Answer from the drawing. Dimensions are ordinates in mm from the lowest x, y and z of the part. A direction names the side the tool comes from. Give positions to 0.01 mm unless a question says otherwise; leave off trailing zeros. Loops run counter-clockwise (first coordinate to the right, second up) from the corner with the lowest first, then second, coordinate; pieces in that order, holes last. Notation, with made-up numbers: (-8, 45.5) - (47, 45.5) arc R15 ccw to (47, 69.5) - close; hole circle Ø9 at (20, 69). An arc over 180 degrees is marked (long way). Answer as CSV lines item,"result". Start each with the question number.
1) Flat-ended cylindrical pins translate along their axes: pin 1 (1.5 mm diameter, centred on x = 3.5, y = 1.5, fed in from +Z); pin 2 (1.5 mm diameter, centred on y = 5, z = 6.5, fed in from -X); pin 3 (1 mm diameter, centred on y = 1.5, z = 3, fed in from -X). Find the tip coordinate at first contact, or state that the pin passes through.
2) A cutting plane is placed at B-B (x = 10). Determine the outline of the cut face in (y, z), and give its area (3 significant figures).
3) For a pull along X with two mould halves and no side action, classify the marked faces 1, 2 and 3 as pulls with the +X half, pulls with the -X half, needs draft (parallel to the pull), parting line crosses it, or undercut.
4) A cutting plane is placed at A-A (z = 10). Determine the outline of the cut face in (x, y), and give its area (3 significant figures).
5) Find the intervals of material crossed by line 1 along X through (y, z) = (3, 10); line 2 along Y through (x, z) = (3.5, 8.5); line 3 along Z through (x, y) = (11.25, 5.5), in increasing order.
6) A cutting plane is placed at C-C (y = 2). Determine the outline of the cut face in (x, z).
7) For the marked faces 4, 5 and 6, determine the directions among +Z, -Z, +X, -X, +Y, -Y from which every point of the face is accessible in a straight line to the end or side of a thin tool.
8) A cutting plane is placed at D-D (z = 4.25). Determine the outline of the cut face in (x, y), and give its area (3 significant figures).
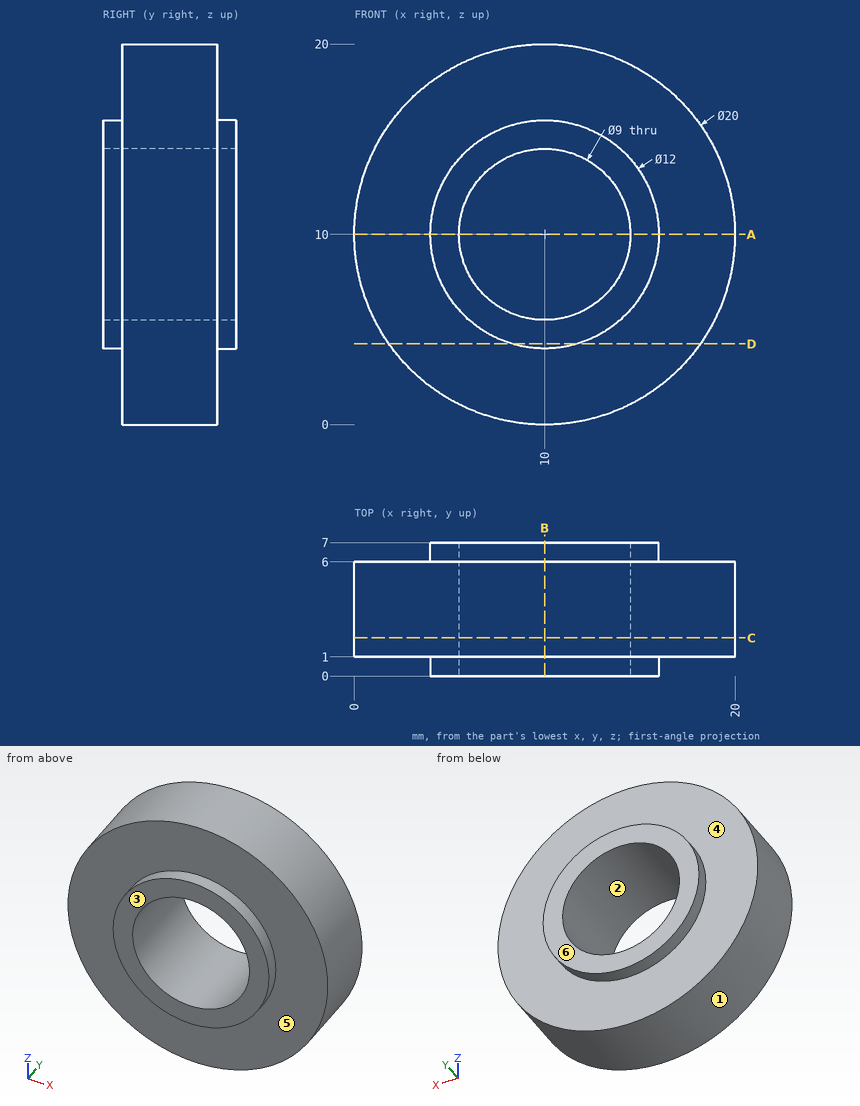
Ans:
1,pin 1,"z = 18.18"
1,pin 2,"x = 0.39"
1,pin 3,"x = 2.4"
2,outline,"(0, 4) - (1, 4) - (1, 0) - (6, 0) - (6, 4) - (7, 4) - (7, 5.5) - (0, 5.5) - close; (0, 14.5) - (7, 14.5) - (7, 16) - (6, 16) - (6, 20) - (1, 20) - (1, 16) - (0, 16) - close"
2,area,"61.0 mm2"
3,face 1,"parting line crosses it"
3,face 2,"undercut"
3,face 3,"needs draft"
4,outline,"(0, 1) - (4, 1) - (4, 0) - (5.5, 0) - (5.5, 7) - (4, 7) - (4, 6) - (0, 6) - close; (14.5, 0) - (16, 0) - (16, 1) - (20, 1) - (20, 6) - (16, 6) - (16, 7) - (14.5, 7) - close"
4,area,"61.0 mm2"
5,line 1,"0 to 5.5, 14.5 to 20"
5,line 2,"1 to 6"
5,line 3,"0.08 to 5.68, 14.32 to 19.92"
6,outline,"circle Ø20 at (10, 10); hole circle Ø9 at (10, 10)"
7,face 4,"+Y"
7,face 5,"-Y"
7,face 6,"+Z, -Z, +X, -X, +Y"
8,outline,"(1.82, 1) - (8.29, 1) - (8.29, 0) - (11.71, 0) - (11.71, 1) - (18.18, 1) - (18.18, 6) - (11.71, 6) - (11.71, 7) - (8.29, 7) - (8.29, 6) - (1.82, 6) - close"
8,area,"88.7 mm2"
